Can you work these out from the model? Positions are in its coordinate system, mm. A direction names the side the tool comes from. Round coordinates to 2 decimals unless told otherwise and drop trailing zeros. Order: outer loops, then holes, each group sorted by start corner. A loop starts at its lowest first (then second) coordinate and runs counter-clockwise, first axis right, second up. Notation, with made-up numbers: (37, -2.5) -> (82, -2.5) arc R27 ccw to (82, 24.5) -> close; hole circle Ø9 at (-28, 63). An arc over 180 degrees is marked (long way). Use a Markdown table: item, result. Add a question column.
Q1. If we section it at B-B on x = 1: List the corners of the cut face in (y, z) for me, plus the area to 3 significant figures.
Q2. If we section it at A-A on y = 35: List the corners of the cut face in (x, z) for me.
Q3. I'm going to push flat-ended pins straight in: pin 1 Ø11 at (x, y) = (-22.5, 11.5) entering from -Z; pin 2 Ø3.5 at (x, y) = (-24.5, 46.97) entering from -Z; pin 3 Ø5.5 at (x, y) = (-28.86, -7.59) entering from +Z; pin 4 Ø8 at (x, z) = (25, -14.5) entering from +Y. Where does each tip first touch, or does it pass through?
Q4. I need wall thicknesses on line 1 along Y through (x, z) = (1, -7.5); line 2 along Y through (x, z) = (24.5, 0.8); line 3 along Y through (x, z) = (-21, 1.55). Which ranges of each line are inside material? Lowest first, please. Write a range as [from, to].
Q5. If we section it at D-D on y = 21.5: List the corners of the cut face in (x, z) for me.
Q6. We'd pull the mould along Z, two halves only. Please class faces 3 (the face through (-20.2, -22.7, 1)), 4 (the face through (-29.809, 0.801, -9.317)), 5 (the face through (-14.6, -26.2, -9)), 6 (the face through (-7, 16, 0)): +Z half, -Z half, draft (parallel to the pull), parting line (faces both ways), or undercut.
Q7. If we section it at C-C on x = 20.5: List the corners of the cut face in (y, z) for me.
Q8. For faces 1 (the face through (0, -27.202, -12)), 2 (the face through (-16, -12.702, 1)), which set-ups out of +Z, -Z, +X, -X, +Y, -Y let a thin tool reach every point of the face, with its end or its side?
```python
from build123d import *

# Parameters (mm, degrees)
PAD_DEPTH       = 47
SKETCH002_R     = 1.7
SKETCH002_R_2   = 1.5
PAD001_DEPTH    = 2
PAD002_DEPTH    = 2
SKETCH004_R     = 1.75
SKETCH004_W     = 23.5
SKETCH004_H     = 32.75
POCKET_DEPTH    = 2
SKETCH005_R     = 1.75
SKETCH005_W     = 23.5
SKETCH005_H     = 32.75
POCKET001_DEPTH = 2
SKETCH006_R     = 1.75
SKETCH006_W     = 23.5
SKETCH006_H     = 32.75
POCKET002_DEPTH = 2
SKETCH007_W     = 4
SKETCH007_H     = 13.3147552139
PAD003_DEPTH    = 2
PAD004_DEPTH    = 3
PAD005_DEPTH    = 3
PAD006_DEPTH    = 4


with BuildPart() as part:
    # Sketch (on XY_Plane of Origin) → Pad (new body)
    with BuildSketch(Plane.XY):
        Polygon((-11.9800180857, 33.6534118443), (11.9800180857, 33.6534118443), (35.1347186241, -6.4517059222), (23.1547005384, -27.2017059222), (-23.1547005384, -27.2017059222), (-35.1347186241, -6.4517059222), align=None)
        Polygon((-10.8253175473, 31.6534118443), (10.8253175473, 31.6534118443), (32.8253175473, -6.4517059222), (22, -25.2017059222), (-22, -25.2017059222), (-32.8253175473, -6.4517059222), align=None, mode=Mode.SUBTRACT)
    extrude(amount=-PAD_DEPTH)

    # Sketch002 (on Face13 of Pad) → Pad001 (join)
    with BuildSketch(Plane.XY):
        with BuildLine():
            ThreePointArc((-22.9999999997, 44.3700908485), (-21.9019237891, 45.4681670596), (-21.5000000007, 46.9681670589))
            Line((-21.5000000007, 46.9681670582), (21.5, 46.9681670582))
            ThreePointArc((21.5, 46.9681670589), (26.6212972707, 44.8468236428), (24.5000652595, 49.9681670582))
            Line((24.5000652595, 49.9681670582), (-24.5, 49.9681670582))
            ThreePointArc((-24.5, 49.9681670582), (-27.0980762107, 48.4681670586), (-27.0980762107, 45.4681670593))
            Line((-27.0980762107, 45.4681670593), (-16.1284210963, 26.4681670596))
            Line((-16.1284210963, 26.4681670596), (-35.1347186241, -6.4517059222))
            Line((-35.1347186241, -6.4517059222), (-23.1547005384, -27.2017059222))
            Line((-23.1547005384, -27.2017059222), (23.1547005384, -27.2017059222))
            Line((23.1547005384, -27.2017059222), (35.1347186241, -6.4517059222))
            Line((35.1347186241, -6.4517059222), (11.9800180857, 33.6534118443))
            Line((11.9800180857, 33.6534118443), (-11.9800180857, 33.6534118443))
            Line((-11.9800180857, 33.6534118443), (-14.3963702888, 29.4681670596))
            Line((-14.3963702888, 29.4681670596), (-22.9999999997, 44.3700908485))
        make_face()
        Polygon((6, 15.0111069989), (0, 25.4034118443), (-6, 15.0111069989), (-13.3612159322, 19.2611069989), (-23.3612159322, 1.9405989232), (-16, -2.3094010768), (-22, -12.7017059222), (-10, -12.7017059222), (-10, -21.2017059222), (10, -21.2017059222), (10, -12.7017059222), (22, -12.7017059222), (16, -2.3094010768), (23.3612159322, 1.9405989232), (13.3612159322, 19.2611069989), align=None, mode=Mode.SUBTRACT)
        with Locations((-7.8612159322, 28.7873864406)):
            Circle(SKETCH002_R, mode=Mode.SUBTRACT)
        with Locations((-28.8612159322, -7.5856805184)):
            Circle(SKETCH002_R, mode=Mode.SUBTRACT)
        with Locations((7.8612159322, 28.7873864406)):
            Circle(SKETCH002_R, mode=Mode.SUBTRACT)
        with Locations((28.8612159322, -7.5856805184)):
            Circle(SKETCH002_R, mode=Mode.SUBTRACT)
        with Locations((-21, -21.2017059222)):
            Circle(SKETCH002_R, mode=Mode.SUBTRACT)
        with Locations((21, -21.2017059222)):
            Circle(SKETCH002_R, mode=Mode.SUBTRACT)
        with Locations((24.5, 46.9681670589)):
            Circle(SKETCH002_R_2, mode=Mode.SUBTRACT)
        with Locations((-24.5, -11.0318329411)):
            Circle(SKETCH002_R_2, mode=Mode.SUBTRACT)
        with Locations((24.5, -11.0318329411)):
            Circle(SKETCH002_R_2, mode=Mode.SUBTRACT)
        with Locations((-24.5, 46.9681670589)):
            Circle(SKETCH002_R_2, mode=Mode.SUBTRACT)
    extrude(amount=PAD001_DEPTH)

    # Sketch003 (on Face9 of Pad001) → Pad002 (join)
    with BuildSketch(Plane(origin=(0, 0, 0), x_dir=(1, 0, 0), z_dir=(0, 0, -1))):
        Polygon((16.1284210968, -26.4681670589), (27.0980762114, -45.4681670589), (23, -44.3700908476), (14.3963702892, -29.4681670589), align=None)
    extrude(amount=-PAD002_DEPTH)

    # Sketch004 (on Face5 of Pad002) → Pocket (cut)
    with BuildSketch(Plane.XZ.offset(27.2017059222)):
        with Locations((15.5, -10.5)):
            Circle(SKETCH004_R)
        with Locations((-15.5, -10.5)):
            Circle(SKETCH004_R)
        with Locations((-15.5, -41.5)):
            Circle(SKETCH004_R)
        with Locations((15.5, -41.5)):
            Circle(SKETCH004_R)
        with Locations((0, -30.625)):
            Rectangle(SKETCH004_W, SKETCH004_H)
    extrude(amount=-POCKET_DEPTH, mode=Mode.SUBTRACT)

    # Sketch005 (on Face3 of Pocket) → Pocket001 (cut)
    with BuildSketch(Plane(origin=(23.5573683549, 13.6008529611, 0), x_dir=(-0.5, 0.8660254038, 0), z_dir=(0.8660254038, 0.5, 0))):
        with Locations((15.5, -10.5)):
            Circle(SKETCH005_R)
        with Locations((-15.5, -10.5)):
            Circle(SKETCH005_R)
        with Locations((-15.5, -41.5)):
            Circle(SKETCH005_R)
        with Locations((15.5, -41.5)):
            Circle(SKETCH005_R)
        with Locations((0, -30.625)):
            Rectangle(SKETCH005_W, SKETCH005_H)
    extrude(amount=-POCKET001_DEPTH, mode=Mode.SUBTRACT)

    # Sketch006 (on Face13 of Pocket001) → Pocket002 (cut)
    with BuildSketch(Plane(origin=(-23.5573683549, 13.6008529611, 0), x_dir=(-0.5, -0.8660254038, 0), z_dir=(-0.8660254038, 0.5, 0))):
        with Locations((15.5, -10.5)):
            Circle(SKETCH006_R)
        with Locations((-15.5, -10.5)):
            Circle(SKETCH006_R)
        with Locations((-15.5, -41.5)):
            Circle(SKETCH006_R)
        with Locations((15.5, -41.5)):
            Circle(SKETCH006_R)
        with Locations((0, -30.625)):
            Rectangle(SKETCH006_W, SKETCH006_H)
    extrude(amount=-POCKET002_DEPTH, mode=Mode.SUBTRACT)

    # Sketch007 (on Face10 of Pocket002) → Pad003 (join)
    with BuildSketch(Plane.XY.offset(2)):
        with Locations((0, 40.3107894513)):
            Rectangle(SKETCH007_W, SKETCH007_H)
    extrude(amount=-PAD003_DEPTH)

    # Sketch008 (on Face17 of Pad003) → Pad004 (join)
    with BuildSketch(Plane(origin=(-1.9628129211, 1.1332305684, 0), x_dir=(-0.5, -0.8660254038, 0), z_dir=(-0.8660254038, 0.5, 0))):
        Polygon((-49.9256258422, 0), (-30.986315613, 0), (-30.986315613, -5), align=None)
    extrude(amount=-PAD004_DEPTH)

    # Sketch009 (on Face34 of Pad004) → Pad005 (join)
    with BuildSketch(Plane(origin=(1.9628129217, 1.1332305687, 0), x_dir=(-0.5, 0.8660254038, 0), z_dir=(0.8660254038, 0.5, 0))):
        Polygon((49.9256258429, 0), (30.9863156134, 0), (30.9863156134, -5), align=None)
    extrude(amount=-PAD005_DEPTH)

    # Sketch010 (on Face13 of Pad005) → Pad006 (join)
    with BuildSketch(Plane(origin=(-2, 0, 0), x_dir=(0, -1, 0), z_dir=(-1, 0, 0))):
        Polygon((-46.9681670582, 0), (-33.6534118443, 0), (-33.6534118443, -5), align=None)
    extrude(amount=-PAD006_DEPTH)


solid = part.part
```
Answer below:
| question | item | result |
|---|---|---|
| 1 | outline | (-27.2, -14.25) -> (-25.2, -14.25) -> (-25.2, 0) -> (-21.2, 0) -> (-21.2, 2) -> (-27.2, 2) -> close; (23.67, 0) -> (31.65, 0) -> (31.65, -47) -> (33.65, -47) -> (33.65, -5) -> (46.97, 0) -> (49.97, 0) -> (49.97, 2) -> (23.67, 2) -> close |
| 1 | area | 220 mm² |
| 2 | outline | (-21.05, -2.4) -> (-17.59, -2.86) -> (-17.59, 2) -> (-21.05, 2) -> close; (-2, -4.49) -> (2, -4.49) -> (2, 2) -> (-2, 2) -> close; (17.59, -2.86) -> (21.05, -2.4) -> (21.05, 2) -> (17.59, 2) -> close |
| 3 | pin 1 | z = -14.25 |
| 3 | pin 2 | z = 0 |
| 3 | pin 3 | z = 2 |
| 3 | pin 4 | y = 18.02 |
| 4 | line 1 | [-27.2, -25.2], [31.65, 33.65] |
| 4 | line 2 | [-24.87, -12.53], [-9.53, 11.97], [40.97, 45.47], [48.47, 49.97] |
| 4 | line 3 | [-27.2, -22.9], [-19.5, -12.7], [-10.97, 0.58], [6.03, 18.03], [34.91, 40.91], [46.97, 49.97] |
| 5 | outline | (-19, -14.25) -> (-16.69, -14.25) -> (-16.69, 0) -> (-2.25, 0) -> (-2.25, 2) -> (-19, 2) -> close; (2.25, 0) -> (16.69, 0) -> (16.69, -14.25) -> (19, -14.25) -> (19, 2) -> (2.25, 2) -> close |
| 6 | face 3 | draft |
| 6 | face 4 | undercut |
| 6 | face 5 | undercut |
| 6 | face 6 | -Z half |
| 7 | outline | (-27.2, -47) -> (-25.2, -47) -> (-25.2, 0) -> (-22.83, 0) -> (-22.83, 2) -> (-27.2, 2) -> close; (-19.58, 0) -> (-12.7, 0) -> (-12.7, 2) -> (-19.58, 2) -> close; (-10.1, 0) -> (0.29, 0) -> (0.29, 2) -> (-10.1, 2) -> close; (6.9, 0) -> (14.9, 0) -> (14.9, -14.25) -> (18.9, -14.25) -> (18.9, 2) -> (6.9, 2) -> close; (34.04, -2.69) -> (40.04, -1.32) -> (40.04, 2) -> (34.04, 2) -> close; (46.97, 0) -> (49.97, 0) -> (49.97, 2) -> (46.97, 2) -> close |
| 8 | face 1 | +Z, -Z, +X, -X, -Y |
| 8 | face 2 | +Z, -Z |
